Build history of the part. All positions in model axes, mm. Face numbers are marked on the shaded views. A direction names the side the tool comes from. Round coordinates to 2 decimals unless told otherwise and drop trailing zeros. Write each loop counter-clockwise with the first axis right and the second up, starting at its lowest first coordinate (ties: lowest second). Pieces come first, ordered by that corner, then holes.
Item 1: Band-saw the part on C-C, the plane y = -36.45. Write the cut outline in (x, z), then the cut area to 3 significant figures.
Item 2: Wall check: probe 1 along Y at (x, z) = (0, -20.6) (3 decimals); probe 2 along X at (y, z) = (-17, -9.25); probe 3 along Y at (x, z) = (5.5, -1.5). Give the ranges that are in metal, low to high.
Item 3: Band-saw the part on B-B, the plane z = -11.25. Write the cut outline in (x, y).
Item 4: 3-axis set-ups, long thin cutter, end or side, ignore diameter. For the marked faces 1 and 2: which of +Z, -Z, +X, -X, +Y, -Y reach the whole face in a straight line?
Item 5: Drop flat-ended pins along their axis: pin 1 Ø1.1 at (x, y) = (-10, 16) entering from +Z; pin 2 Ø0.8 at (x, y) = (-10, 28) entering from +Z; pin 3 Ø0.5 at (x, y) = (-10, 1) entering from +Z; pin 4 Ø1.5 at (y, z) = (11, -5) entering from -X. Give the stop position or say it passes through.
Item 6: Mould opens along Y. For the marked faces 3, 4 and 5 say: +Y half, -Y half, draft (parallel to the pull), parting line (faces both ways), or undercut.
Item 7: Band-saw the part on D-D, the plane z = -15.5. Write the cut outline in (x, y), then the cut area to 3 significant figures.
Item 8: Band-saw the part on A-A, the plane x = 0. Write the cut outline in (y, z) (3 decimals), then the cut area to 3 significant figures.
```python
from build123d import *

# Parameters (mm, degrees)
SKETCH1_W           = 20.9
SKETCH1_H           = 21.4
BOSS_EXTRUDE1_DEPTH = 38.85
SKETCH2_W           = 18.9
SKETCH2_H           = 75.7
CUT_EXTRUDE1_DEPTH  = 20.4
CUT_EXTRUDE4_DEPTH  = 50.031545968
SKETCH4_R           = 1.2
BOSS_EXTRUDE2_DEPTH = 2
SKETCH5_R           = 1.6
CUT_EXTRUDE5_DEPTH  = 46.568464973
FILLET1_R           = 3


with BuildPart() as part:
    # Sketch1 → Boss-Extrude1 (new, symmetric)
    with BuildSketch(Plane(origin=(0, 0, 0), x_dir=(1, 0, 0), z_dir=(0, 1, 0))):
        with Locations((0, 10.7)):
            Rectangle(SKETCH1_W, SKETCH1_H)
    extrude(amount=BOSS_EXTRUDE1_DEPTH, both=True)

    # Sketch2 → Cut-Extrude1 (cut)
    with BuildSketch(Plane(origin=(0, 0, 0), x_dir=(-1, 0, 0), z_dir=(0, 0, -1))):
        Rectangle(SKETCH2_W, SKETCH2_H)
    extrude(amount=CUT_EXTRUDE1_DEPTH, mode=Mode.SUBTRACT)

    # Sketch3 → Cut-Extrude4 (cut, through all)
    with BuildSketch(Plane(origin=(10.45, 0, 0), x_dir=(0, 0, -1), z_dir=(1, 0, 0))):
        Polygon((0, 37.85), (3, 37.85), (3, 22.85), (7, 18.472222222), (7, 11.472222222), (12, 6), (12, -6), (7, -11.472222222), (7, -18.472222222), (3, -22.85), (3, -37.85), (0, -37.85), align=None)
    extrude(amount=-CUT_EXTRUDE4_DEPTH, mode=Mode.SUBTRACT)

    # Sketch4 → Boss-Extrude2 (add)
    with BuildSketch(Plane(origin=(0, 0, -21.4), x_dir=(-1, 0, 0), z_dir=(0, 0, -1))):
        with Locations(Location((0, -36.45, 0), (0, 0, 180))):
            Circle(SKETCH4_R)
        with Locations(Location((0, 36.45, 0), (0, 0, 180))):
            Circle(SKETCH4_R)
    extrude(amount=BOSS_EXTRUDE2_DEPTH)

    # Sketch5 → Cut-Extrude5 (cut, through all)
    with BuildSketch(Plane(origin=(0, 0, -21.4), x_dir=(-1, 0, 0), z_dir=(0, 0, -1))):
        with Locations((0, -27.805)):
            Circle(SKETCH5_R)
        with Locations(Location((0, 27.805, 0), (0, 0, 180))):
            Circle(SKETCH5_R)
    extrude(amount=-CUT_EXTRUDE5_DEPTH, mode=Mode.SUBTRACT)

    # Fillet1
    fillet1_edges = [part.edges().sort_by_distance(p)[0] for p in [
        (-10.45, 38.35, 0),
        (10.45, 38.35, 0),
        (-10.45, -38.35, 0),
        (10.45, -38.35, 0),
    ]]
    fillet(fillet1_edges, radius=FILLET1_R)


solid = part.part
```
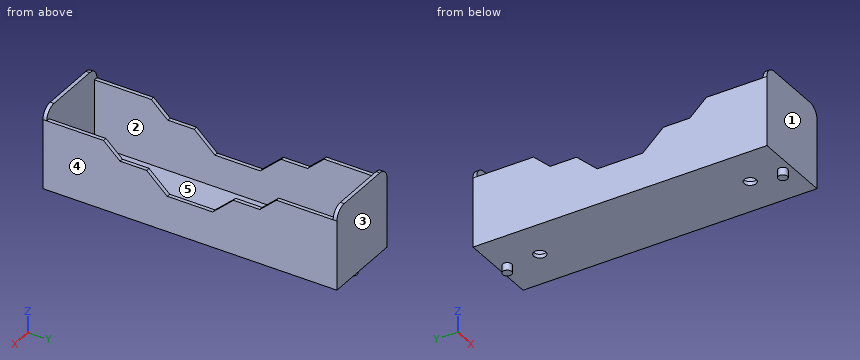
Results:
1. outline: (-10.45, -21.4) - (-1.2, -21.4) - (-1.2, -23.4) - (1.2, -23.4) - (1.2, -21.4) - (10.45, -21.4) - (10.45, -3) - (9.45, -3) - (9.45, -20.4) - (-9.45, -20.4) - (-9.45, -3) - (-10.45, -3) - close
1. area: 60.5 mm2
2. probe 1: y = -38.85 to -29.405, -26.205 to 26.205, 29.405 to 38.85
2. probe 2: x = -10.45 to -9.45, 9.45 to 10.45
2. probe 3: y = -38.85 to -37.85, 37.85 to 38.85
3. outline: (-10.45, -38.85) - (10.45, -38.85) - (10.45, -6.82) - (9.45, -6.82) - (9.45, -37.85) - (-9.45, -37.85) - (-9.45, -6.82) - (-10.45, -6.82) - close; (-10.45, 6.82) - (-9.45, 6.82) - (-9.45, 37.85) - (9.45, 37.85) - (9.45, 6.82) - (10.45, 6.82) - (10.45, 38.85) - (-10.45, 38.85) - close
4. face 1: +Z, -Z, +X, -X, -Y
4. face 2: +Z
5. pin 1: stops at z = -7
5. pin 2: stops at z = -3
5. pin 3: stops at z = -12
5. pin 4: passes through
6. face 3: +Y half
6. face 4: draft
6. face 5: undercut
7. outline: (-10.45, -38.85) - (10.45, -38.85) - (10.45, 38.85) - (-10.45, 38.85) - close; hole (-9.45, -37.85) - (9.45, -37.85) - (9.45, 37.85) - (-9.45, 37.85) - close
7. area: 193 mm2
8. outline: (-38.85, -21.4) - (-37.65, -21.4) - (-37.65, -23.4) - (-35.25, -23.4) - (-35.25, -21.4) - (-29.405, -21.4) - (-29.405, -20.4) - (-37.85, -20.4) - (-37.85, 0) - (-38.85, 0) - close; (-26.205, -21.4) - (26.205, -21.4) - (26.205, -20.4) - (-26.205, -20.4) - close; (29.405, -21.4) - (35.25, -21.4) - (35.25, -23.4) - (37.65, -23.4) - (37.65, -21.4) - (38.85, -21.4) - (38.85, 0) - (37.85, 0) - (37.85, -20.4) - (29.405, -20.4) - close
8. area: 122 mm2
